The figure shows three views and two pictorial views of one solid part (mm, origin at its lowest corner). Answer the questions. A direction names the side the tool comes from. Round coordinates to 2 decimals unless told otherwise and drop trailing zeros. Write each loop counter-clockwise with the first axis right and the second up, starting at its lowest first coordinate (ties: lowest second). Pieces come first, ordered by that corner, then holes. Notation, with made-up numbers: (58, 27) - (75, 27) arc R15 ccw to (75, 47) - close; hole circle Ø4 at (-37.5, 4). An arc over 180 degrees is marked (long way). Answer as CSV lines item,"result". Start each with the question number.
Item 1: Flat-ended cylindrical pins translate along their axes: pin 1 (1 mm diameter, centred on x = 15, z = 10, fed in from -Y); pin 2 (13 mm diameter, centred on y = 43, z = 19.5, fed in from -X); pin 3 (11 mm diameter, centred on y = 73, z = 16, fed in from +X). Find the tip coordinate at first contact, or state that the pin passes through.
Item 2: A cutting plane is placed at A-A on x = 2. Determine the outline of the cut face in (y, z), and give its area (3 significant figures).
Item 3: Which of the six approach directions +Z, -Z, +X, -X, +Y, -Y give full straight-line access (tool end or side, diameter ignored) to the marked faces 1, 2 and 3?
Item 4: Straight lines are drawn through the part: line 1 along Z through (x, y) = (4.25, 77); line 2 along Y through (x, z) = (8.75, 15); line 3 along X through (y, z) = (59, 14). For each, find the intervals that lie inside material, in ascending order. Write a range as [from, to].
Item 5: A cutting plane is placed at B-B on y = 45.5. Determine the outline of the cut face in (x, z) (1 decimal).
Item 6: A cutting plane is placed at C-C on z = 15. Determine the outline of the cut face in (x, y) (1 decimal).
Item 7: For a pull along Y with two mould halves and no side action, classify the marked faces 4, 5, 6 and 7 as pulls with the +Y half, pulls with the -Y half, needs draft (parallel to the pull), parting line crosses it, or undercut.
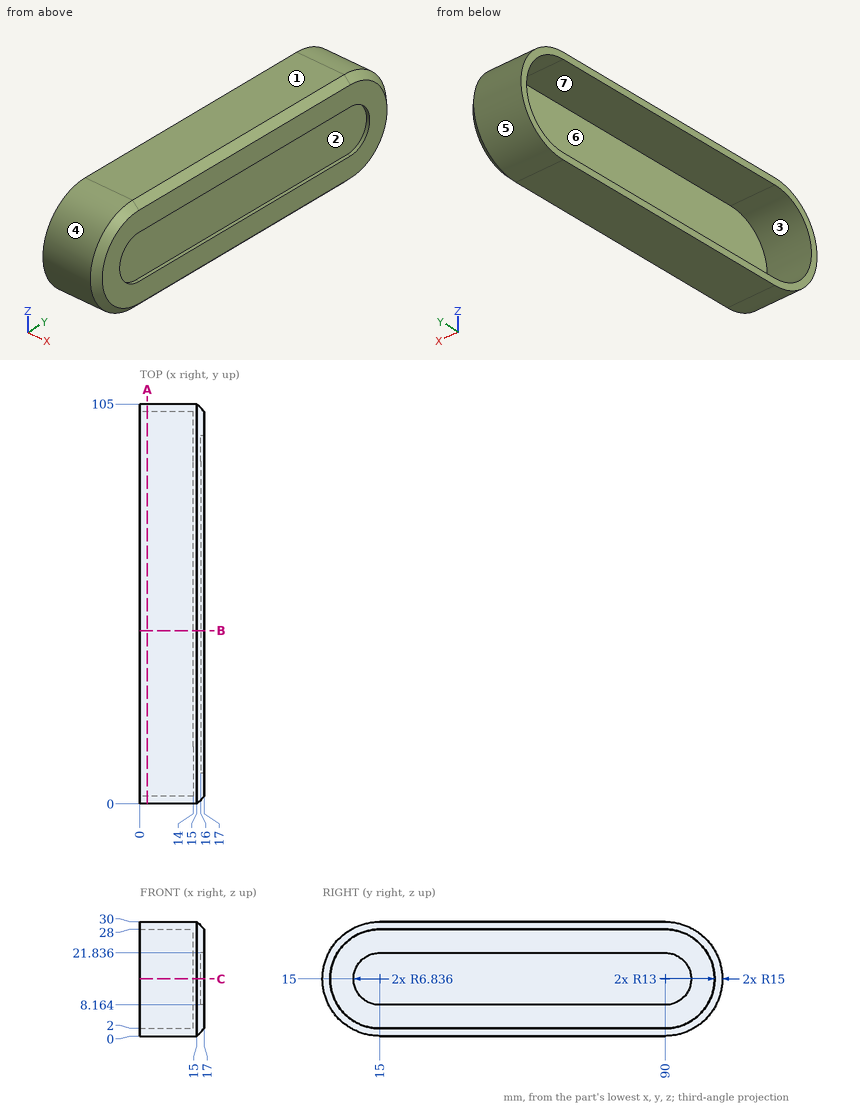
Geometry says:
1,pin 1,"stops at y = 0.69"
1,pin 2,"stops at x = 14"
1,pin 3,"stops at x = 16"
2,outline,"(15, 0) - (90, 0) arc R15 ccw to (90, 30) - (15, 30) arc R15 ccw to start; hole (15, 2) - (90, 2) arc R13 ccw to (90, 28) - (15, 28) arc R13 ccw to start"
2,area,"476 mm^2"
3,face 1,"+Z, +X, -X, +Y, -Y"
3,face 2,"+X"
3,face 3,"-X"
4,line 1,"z = [0, 2], [28, 30]"
4,line 2,"y = [0, 2], [103, 105]"
4,line 3,"x = [14, 16]"
5,outline,"(0, 0) - (15, 0) - (17, 2) - (17, 8.2) - (16, 8.2) - (16, 21.8) - (17, 21.8) - (17, 28) - (15, 30) - (0, 30) - (0, 28) - (14, 28) - (14, 2) - (0, 2) - close"
6,outline,"(0, 0) - (15, 0) - (17, 2) - (17, 8.2) - (16, 8.2) - (16, 96.8) - (17, 96.8) - (17, 103) - (15, 105) - (0, 105) - (0, 103) - (14, 103) - (14, 2) - (0, 2) - close"
7,face 4,"pulls with the -Y half"
7,face 5,"pulls with the +Y half"
7,face 6,"undercut"
7,face 7,"undercut"
